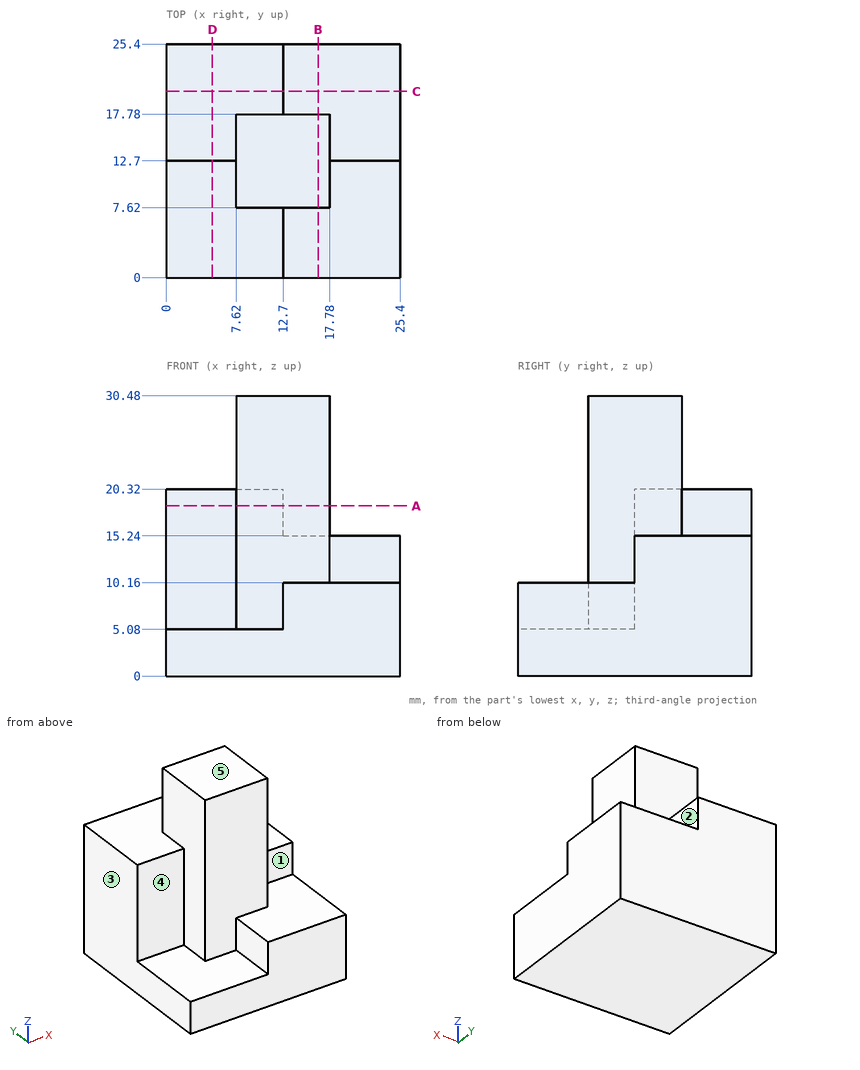
Design review of the part shown in the three views and the two pictorial views. Dimensions are in mm from the part's minimum x, y and z. A direction names the side the tool comes from. Round coordinates to 2 decimals unless told otherwise and drop trailing zeros. Loops run counter-clockwise (first coordinate to the right, second up) from the corner with the lowest first, then second, coordinate; pieces in that order, holes last. Notation, with made-up numbers: M 31,-12 L 86,-12 A24 cw 86,26 Z; hole C 27.25,51.25 d9. An arc over 180 degrees is marked long. Answer as a JSON object with one key per item and string values.
Item 1: Tool access review of the marked faces 1, 2, 3, 4 and 5: name each direction out of +Z, -Z, +X, -X, +Y, -Y from which nothing blocks a thin tool from reaching the whole face with its end or side.
Check sheet entries:
{"face 1": "+Z, +X, -Y", "face 2": "+Z, +X, +Y", "face 3": "+Z, -Z, -X, +Y, -Y", "face 4": "+Z, -X, -Y", "face 5": "+Z, +X, -X, +Y, -Y"}
Item 2: We need section C-C, the plane y = 20.25. State the section outline as (x, z) points.
Check sheet entries:
{"outline": "M 0,0 L 25.4,0 L 25.4,15.24 L 12.7,15.24 L 12.7,20.32 L 0,20.32 Z"}
Item 3: We need section D-D, the plane x = 5. State the section outline as (y, z) points.
Check sheet entries:
{"outline": "M 0,0 L 25.4,0 L 25.4,20.32 L 12.7,20.32 L 12.7,5.08 L 0,5.08 Z"}
Item 4: We need section B-B, the plane x = 16.5. State the section outline as (y, z) points.
Check sheet entries:
{"outline": "M 0,0 L 25.4,0 L 25.4,15.24 L 17.78,15.24 L 17.78,30.48 L 7.62,30.48 L 7.62,10.16 L 0,10.16 Z"}
Item 5: We need section A-A, the plane z = 18.5. State the section outline as (x, y) points.
Check sheet entries:
{"outline": "M 0,12.7 L 7.62,12.7 L 7.62,7.62 L 17.78,7.62 L 17.78,17.78 L 12.7,17.78 L 12.7,25.4 L 0,25.4 Z"}
Item 6: Clearance check with flat-ended pins moving along their axes: P1, Ø5, axis at x = 14, z = 25, coming from the +Y side; P2, Ø8, axis at x = 13, z = 20, coming from the -Y side; P3, Ø4, axis at x = 15.5, y = 17, coming from the -Z side; P4, Ø1.5, axis at y = 21, z = 18, coming from the +X side. State where each tip first meets the part, or that it passes through.
Check sheet entries:
{"P1": "y = 17.78", "P2": "y = 7.62", "P3": "z = 0", "P4": "x = 12.7"}
Item 7: For line 1 along Z through (x, y) = (12.25, 19.5); line 2 along Z through (x, y) = (3.25, 4); line 3 along X through (y, z) = (5.5, 9), list the stretches that pass through material, from the lowest coordinate up.
Check sheet entries:
{"line 1": "0 to 20.32", "line 2": "0 to 5.08", "line 3": "12.7 to 25.4"}
